Design review of the part built by this model. Coordinates are the model's own, in mm. Face numbers are marked on the shaded views. A direction names the side the tool comes from. Round coordinates to 2 decimals unless told otherwise and drop trailing zeros. Loops run counter-clockwise (first coordinate to the right, second up) from the corner with the lowest first, then second, coordinate; pieces in that order, holes last. Notation, with made-up numbers: (46, -27) -> (95, -27) arc R8 cw to (95, -14) -> close; hole circle Ø7 at (0, 83). An arc over 180 degrees is marked (long way). Write each question's results on one line, items separated by ' | '. Start each with the question number.
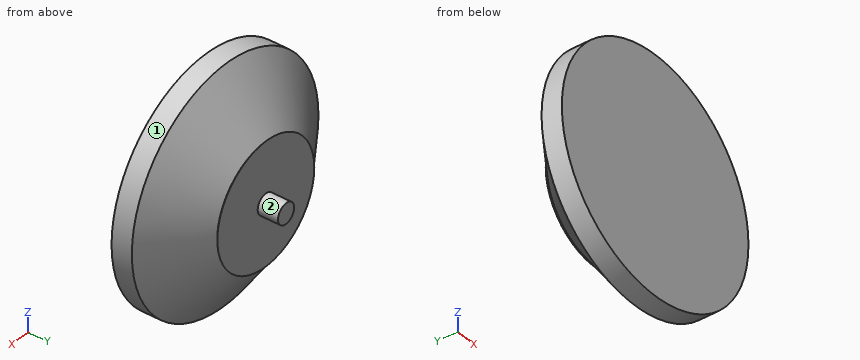
from build123d import *

# Parameters (mm, degrees)
SKETCH11_R          = 12
BOSS_EXTRUDE3_DEPTH = 2
SKETCH13_R          = 11.54797541
BOSS_EXTRUDE4_DEPTH = 2
SKETCH14_R          = 1
BOSS_EXTRUDE5_DEPTH = 2


with BuildPart() as part:
    # Sketch1 → Revolve1 (revolve)
    with BuildSketch(Plane.XY):
        Polygon((0.388993331, -0.067795133), (-5.226777212, -4), (6.321198199, -4), (6.321198199, 6), (-5.678801801, 6), align=None)
    revolve(axis=Axis((6.321198199, 11.047707555, 0), (0, -1, 0)))


with BuildPart() as body_2:
    # Split2: the piece on the far side of the plane
    add(part.part)
    split(bisect_by=Plane.ZX, keep=Keep.BOTTOM)

    # Sketch13 → Boss-Extrude4 (add)
    with BuildSketch(Plane.XZ.offset(4)):
        with Locations((6.321198199, 0)):
            Circle(SKETCH13_R)
    extrude(amount=BOSS_EXTRUDE4_DEPTH)

    # Sketch14 → Boss-Extrude5 (add)
    with BuildSketch(Plane(origin=(0, 0, 0), x_dir=(1, 0, 0), z_dir=(0, 1, 0))):
        with Locations(Location((6.321198199, 0, 0), (0, 0, 270))):
            Circle(SKETCH14_R)
    extrude(amount=BOSS_EXTRUDE5_DEPTH)


with BuildPart() as part_1:
    add(part.part)

    # Split2
    split(bisect_by=Plane.ZX, keep=Keep.TOP)

    # Sketch11 → Boss-Extrude3 (add)
    with BuildSketch(Plane(origin=(0, 6, 0), x_dir=(1, 0, 0), z_dir=(0, 1, 0))):
        with Locations(Location((6.321198199, 0, 0), (0, 0, 180))):
            Circle(SKETCH11_R)
    extrude(amount=BOSS_EXTRUDE3_DEPTH)


solid = body_2.part
1) To check wall thickness, follow line 1 (Y direction, x = 7, z = -5.25); line 2 (Z direction, x = 12, y = -5); line 3 (Z direction, x = -3.25, y = -5.25). State the ranges of each line that lie inside material, in increasing order. Write a range as from..to.
2) Take a section at A-A (z = 0). Write out the cut boundary in (x, y).
3) For the marked faces 1 and 2, list the 3-axis set-ups (+Z, -Z, +X, -X, +Y, -Y) from which the entire face can be reached by the end or side of a thin tool; tool diameter is ignored.
4) Insertion check: pin 1 (3 mm diameter, centred on y = -4.5, z = 3, fed in from +X); pin 2 (4 mm diameter, centred on x = 12.5, z = 5.5, fed in from +Y); pin 3 (6 mm diameter, centred on x = 5.5, z = -9, fed in from +Y); pin 4 (9.5 mm diameter, centred on x = 8.5, z = 2.5, fed in from +Y). Each pin has a flat end and moves straight along its axis. Give the tip position at first contact, or say it passes through.
5) Take a section at B-B (y = -1.5). Write out the cut boundary in (x, z).
Geometry check:
1) line 1: y = -6..0 | line 2: z = -10.06..10.06 | line 3: z = -6.46..6.46
2) outline: (-5.23, -6) -> (17.87, -6) -> (17.87, -4) -> (12.25, -0.07) -> (12.32, 0) -> (7.32, 0) -> (7.32, 2) -> (5.32, 2) -> (5.32, 0) -> (0.32, 0) -> (0.39, -0.07) -> (-5.23, -4) -> close
3) face 1: +Y, -Y | face 2: +Y
4) pin 1: stops at x = 17.77 | pin 2: stops at y = -0.31 | pin 3: stops at y = -0.14 | pin 4: stops at y = 2
5) outline: circle Ø15.96 at (6.32, 0)
